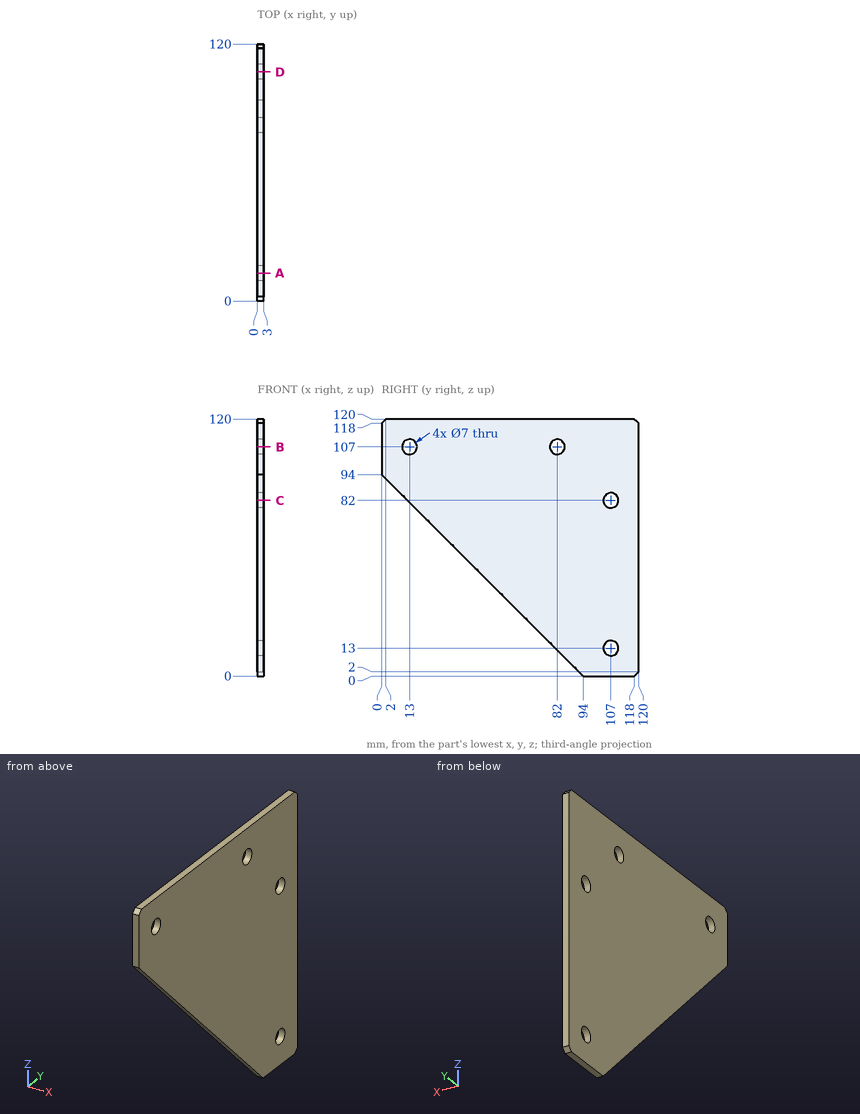
Print and shaded views of the part. All mm, measured from the part's lowest x, y and z. Round coordinates to 2 decimals unless told otherwise and drop trailing zeros. Write each loop counter-clockwise with the first axis right and the second up, starting at its lowest first coordinate (ties: lowest second). Pieces come first, ordered by that corner, then holes.
Item 1: Probe L1, parallel to Z at x = 2.3, y = 107; L2, parallel to Z at x = 1.45, y = 10; L3, parallel to Z at x = 0.6, y = 13. List the from-to ranges inside material, lowest first.
Results:
L1: z = 0 to 9.5, 16.5 to 78.5, 85.5 to 120
L2: z = 84 to 105.2, 108.8 to 120
L3: z = 81 to 103.5, 110.5 to 120
Item 2: Cut at A-A, the plane y = 13. Give the cut face in (x, z).
Results:
outline: (0, 81) - (3, 81) - (3, 103.5) - (0, 103.5) - close; (0, 110.5) - (3, 110.5) - (3, 120) - (0, 120) - close
Item 3: Drop flat-ended pins along their axis: pin 1 Ø1.5 at (x, y) = (2.5, 42) entering from -Z; pin 2 Ø8 at (y, z) = (41, 92.5) entering from -X; pin 3 Ø4 at (y, z) = (82, 107) entering from -X. Give the stop position or say it passes through.
Results:
pin 1: stops at z = 51.25
pin 2: stops at x = 0
pin 3: passes through
Item 4: Cut at B-B, the plane z = 107. Give the cut face in (x, y), plus the area to 3 significant figures.
Results:
outline: (0, 0) - (3, 0) - (3, 9.5) - (0, 9.5) - close; (0, 16.5) - (3, 16.5) - (3, 78.5) - (0, 78.5) - close; (0, 85.5) - (3, 85.5) - (3, 120) - (0, 120) - close
area: 318 mm2
Item 5: Cut at C-C, the plane z = 82. Give the cut face in (x, y), plus the area to 3 significant figures.
Results:
outline: (0, 12) - (3, 12) - (3, 103.5) - (0, 103.5) - close; (0, 110.5) - (3, 110.5) - (3, 120) - (0, 120) - close
area: 303 mm2
